```python
from build123d import *

# Parameters (mm, degrees)
CROQUIS1_W              = 33
CROQUIS1_H              = 33
SALIENTE_EXTRUIR2_DEPTH = 8
VACIADO1_T              = -2
CROQUIS5_W              = 4.422149387
CROQUIS5_H              = 2.5
CORTAR_EXTRUIR3_DEPTH   = 6
CROQUIS6_W              = 32.965049926
CROQUIS6_H              = 12
SALIENTE_EXTRUIR3_DEPTH = 27
CROQUIS7_W              = 32.965049926
CROQUIS7_H              = 2
CORTAR_EXTRUIR4_DEPTH   = 10
CROQUIS8_W              = 10
CROQUIS8_H              = 5
CORTAR_EXTRUIR5_DEPTH   = 10
CROQUIS9_W              = 33
CROQUIS9_H              = 33
CROQUIS9_W_2            = 31
CROQUIS9_H_2            = 31
CORTAR_EXTRUIR6_DEPTH   = 43.065425233


with BuildPart() as part:
    # Croquis1 → Saliente-Extruir2 (new body)
    with BuildSketch(Plane(origin=(0, 0, 0), x_dir=(1, 0, 0), z_dir=(0, 1, 0))):
        Rectangle(CROQUIS1_W, CROQUIS1_H)
    extrude(amount=SALIENTE_EXTRUIR2_DEPTH)

    # Vaciado1
    vaciado1_openings = [part.faces().sort_by_distance(p)[0] for p in [
        (0, 8, 0),
    ]]
    offset(amount=VACIADO1_T, openings=vaciado1_openings, kind=Kind.INTERSECTION)

    # Croquis5 → Cortar-Extruir3 (cut)
    with BuildSketch(Plane(origin=(0, 8, 0), x_dir=(1, 0, 0), z_dir=(0, 1, 0))):
        with Locations((-15.634605234, 0)):
            Rectangle(CROQUIS5_W, CROQUIS5_H)
    extrude(amount=-CORTAR_EXTRUIR3_DEPTH, mode=Mode.SUBTRACT)

    # Croquis6 → Saliente-Extruir3 (add)
    with BuildSketch(Plane.XZ):
        with Locations((0.017475037, 10.5)):
            Rectangle(CROQUIS6_W, CROQUIS6_H)
    extrude(amount=SALIENTE_EXTRUIR3_DEPTH)

    # Croquis7 → Cortar-Extruir4 (cut)
    with BuildSketch(Plane(origin=(0, 0, 4.5), x_dir=(-1, 0, 0), z_dir=(0, 0, -1))):
        with Locations((-0.017475037, -24)):
            Rectangle(CROQUIS7_W, CROQUIS7_H)
        with Locations((-0.017475037, -11)):
            Rectangle(CROQUIS7_W, CROQUIS7_H)
    extrude(amount=-CORTAR_EXTRUIR4_DEPTH, mode=Mode.SUBTRACT)

    # Croquis8 → Cortar-Extruir5 (cut)
    with BuildSketch(Plane(origin=(0, 0, 14.5), x_dir=(-1, 0, 0), z_dir=(0, 0, -1))):
        with Locations((-11.5, -9.5)):
            Rectangle(CROQUIS8_W, CROQUIS8_H)
    extrude(amount=CORTAR_EXTRUIR5_DEPTH, mode=Mode.SUBTRACT)

    # Croquis9 → Cortar-Extruir6 (cut, through all)
    with BuildSketch(Plane(origin=(0, 8, 0), x_dir=(1, 0, 0), z_dir=(0, 1, 0))):
        Rectangle(CROQUIS9_W, CROQUIS9_H)
        Rectangle(CROQUIS9_W_2, CROQUIS9_H_2, mode=Mode.SUBTRACT)
    extrude(amount=-CORTAR_EXTRUIR6_DEPTH, mode=Mode.SUBTRACT)


solid = part.part
```
Work out the finished part from the listing and answer in its coordinate system (mm). A direction names the side the tool comes from. Round coordinates to 2 decimals unless told otherwise and drop trailing zeros. Order: outer loops, then holes, each group sorted by start corner. A loop starts at its lowest first (then second) coordinate and runs counter-clockwise, first axis right, second up.
Q1. A cutting plane is placed at D-D, the plane x = 13. Determine the outline of the cut face in (y, z).
Solution:
outline: (-27, 4.5) - (-25, 4.5) - (-25, 14.5) - (-23, 14.5) - (-23, 4.5) - (-12, 4.5) - (-12, 14.5) - (-7, 14.5) - (-7, 4.5) - (0, 4.5) - (0, -15.5) - (8, -15.5) - (8, -14.5) - (2, -14.5) - (2, 14.5) - (8, 14.5) - (8, 15.5) - (-27, 15.5) - close
Q2. A cutting plane is placed at B-B, the plane y = -9. Determine the outline of the cut face in (x, z), then the cut area to 3 significant figures.
Solution:
outline: (-15.5, 4.5) - (6.5, 4.5) - (6.5, 14.5) - (15.5, 14.5) - (15.5, 15.5) - (-15.5, 15.5) - close
area: 251 mm2
Q3. The mould has two halves that part along Y. Classify faces 1 (the flat face through (0, 0, -6)), 2 (the flat face through (0, 5, 14.5)), 3 (the flat face through (0, -23, 9)): pulls with the +Y half, pulls with the -Y half, needs draft (parallel to the pull), parting line crosses it, or undercut.
Solution:
face 1: pulls with the -Y half
face 2: needs draft
face 3: undercut
Q4. A cutting plane is placed at C-C, the plane z = 4. Determine the outline of the cut face in (x, y), then the cut area to 3 significant figures.
Solution:
outline: (-15.5, 0) - (15.5, 0) - (15.5, 8) - (14.5, 8) - (14.5, 2) - (-14.5, 2) - (-14.5, 8) - (-15.5, 8) - close
area: 74.0 mm2
Q5. Given pin 1 Ø10 at (x, z) = (-11.5, -8.5) entering from -Y; pin 2 Ø1.5 at (x, y) = (7, -10) entering from -Z; pin 3 Ø8.5 at (x, z) = (-6.5, -4) entering from +Y, each flat-ended and moving along its own axis, determine where each tip first touches the part or whether it passes through.
Solution:
pin 1: stops at y = 0
pin 2: stops at z = 4.5
pin 3: stops at y = 2
Q6. A tool of negligible diameter and unlimited length cuts with its end or side. For faces 4 (the flat face through (-15, 5, -1.25)), 5 (the flat face through (6.5, -9, 10)), 6 (the flat face through (0, -26, 4.5)), 7 (the flat face through (0, -24, 14.5)), 8 (the flat face through (-14.5, 5, 8)), from which of +Z, -Z, +X, -X, +Y, -Y can it reach the whole face along a straight path? Write none if from no direction.
Solution:
face 4: -X, +Y
face 5: -Z, +X
face 6: -Z, +X, -X, -Y
face 7: -Z, +X, -X
face 8: +Y
Q7. Find the intervals of material crossed by line 1 along Y through (x, z) = (-7, 8); line 2 along Y through (x, z) = (11.5, 12); line 3 along Z through (x, y) = (8, 4), in increasing order.
Solution:
line 1: y = -27 to -25, -23 to -12, -10 to 2
line 2: y = -27 to -25, -23 to -12, -7 to 2
line 3: z = -15.5 to -14.5, 14.5 to 15.5
Q8. A cutting plane is placed at A-A, the plane x = -5. Determine the outline of the cut face in (y, z).
Solution:
outline: (-27, 4.5) - (-25, 4.5) - (-25, 14.5) - (-23, 14.5) - (-23, 4.5) - (-12, 4.5) - (-12, 14.5) - (-10, 14.5) - (-10, 4.5) - (0, 4.5) - (0, -15.5) - (8, -15.5) - (8, -14.5) - (2, -14.5) - (2, 14.5) - (8, 14.5) - (8, 15.5) - (-27, 15.5) - close
